from build123d import *

# Parameters (mm, degrees)
SKETCH_1_W               = 20
SKETCH_1_H               = 20
SKETCH_1_W_2             = 16
SKETCH_1_H_2             = 16
EXTRUDE_1_DEPTH          = 560
SKETCH_3_R               = 2.2
CUT_EXTRUDE_2_DEPTH      = 560
SKETCH_4_R               = 2.2
CUT_EXTRUDE_3_DEPTH      = 560
SKETCH_7_W               = 41.109335544
SKETCH_7_H               = 41.63539172
CUT_EXTRUDE_7_DEPTH      = 40
SKETCH_8_W               = 53.430317452
SKETCH_8_H               = 33.679555816
CUT_EXTRUDE_8_DEPTH      = 40
SKETCH_9_R               = 1
CUT_EXTRUDE_9_DEPTH      = 10
SKETCH_10_R              = 1
CUT_EXTRUDE_10_DEPTH     = 10
SKETCH_11_R              = 2.1
CUT_EXTRUDE_11_DEPTH     = 21
SKETCH_12_R              = 6
CUT_EXTRUDE_12_DEPTH     = 10
SKETCH_15_R              = 2.1
CUT_EXTRUDE_16_DEPTH     = 21
SKETCH_16_R              = 6
CUT_EXTRUDE_17_DEPTH     = 10
M4X0_7_6_D               = 3.3
M4X0_7_6_DEPTH           = 11.5
M4X0_7_6_TIP             = 0.991420021
M4X0_7_7_D               = 3.3
M4X0_7_7_DEPTH           = 11.5
M4X0_7_7_TIP             = 0.991420021
M4X0_7_7_ON_FACE_2_D     = 3.3
M4X0_7_7_ON_FACE_2_DEPTH = 11.5
M4X0_7_7_ON_FACE_2_TIP   = 0.991420021
SKETCH_26_R              = 1
CUT_EXTRUDE_18_DEPTH     = 10
M4X0_7_9_D               = 3.3
M4X0_7_9_DEPTH           = 11.5
M4X0_7_9_TIP             = 0.991420021


with BuildPart() as part:
    # ｽｹｯﾁ1 → ﾎﾞｽ - 押し出し1 (new body)
    with BuildSketch(Plane.XY):
        Rectangle(SKETCH_1_W, SKETCH_1_H)
        Rectangle(SKETCH_1_W_2, SKETCH_1_H_2, mode=Mode.SUBTRACT)
    extrude(amount=EXTRUDE_1_DEPTH)

    # ｽｹｯﾁ3 → ｶｯﾄ - 押し出し2 (cut)
    with BuildSketch(Plane(origin=(10, 0, 0), x_dir=(0, 0, -1), z_dir=(1, 0, 0))):
        with Locations((-530, 0)):
            Circle(SKETCH_3_R)
        with Locations((-30, 0)):
            Circle(SKETCH_3_R)
    extrude(amount=-CUT_EXTRUDE_2_DEPTH, mode=Mode.SUBTRACT)

    # ｽｹｯﾁ4 → ｶｯﾄ - 押し出し3 (cut)
    with BuildSketch(Plane(origin=(0, 10, 0), x_dir=(1, 0, 0), z_dir=(0, 1, 0))):
        with Locations((0, -550)):
            Circle(SKETCH_4_R)
        with Locations((0, -10)):
            Circle(SKETCH_4_R)
    extrude(amount=-CUT_EXTRUDE_3_DEPTH, mode=Mode.SUBTRACT)

    # ｽｹｯﾁ7 → ｶｯﾄ - 押し出し7 (cut)
    with BuildSketch(Plane(origin=(0, 0, 0), x_dir=(-1, 0, 0), z_dir=(0, 0, -1))):
        Rectangle(SKETCH_7_W, SKETCH_7_H)
    extrude(amount=-CUT_EXTRUDE_7_DEPTH, mode=Mode.SUBTRACT)

    # ｽｹｯﾁ8 → ｶｯﾄ - 押し出し8 (cut)
    with BuildSketch(Plane.XY.offset(560)):
        Rectangle(SKETCH_8_W, SKETCH_8_H)
    extrude(amount=-CUT_EXTRUDE_8_DEPTH, mode=Mode.SUBTRACT)

    # ｽｹｯﾁ9 → ｶｯﾄ - 押し出し9 (cut)
    with BuildSketch(Plane.ZY.offset(10)):
        with Locations((510, 0)):
            Circle(SKETCH_9_R)
        with Locations((490, 0)):
            Circle(SKETCH_9_R)
    extrude(amount=-CUT_EXTRUDE_9_DEPTH, mode=Mode.SUBTRACT)

    # ｽｹｯﾁ10 → ｶｯﾄ - 押し出し10 (cut)
    with BuildSketch(Plane.ZY.offset(10)):
        with Locations((50, 0)):
            Circle(SKETCH_10_R)
        with Locations((70, 0)):
            Circle(SKETCH_10_R)
    extrude(amount=-CUT_EXTRUDE_10_DEPTH, mode=Mode.SUBTRACT)

    # ｽｹｯﾁ11 → ｶｯﾄ - 押し出し11 (cut, through all)
    with BuildSketch(Plane(origin=(0, 10, 0), x_dir=(1, 0, 0), z_dir=(0, 1, 0))):
        with Locations((0, -60)):
            Circle(SKETCH_11_R)
        with Locations((0, -132)):
            Circle(SKETCH_11_R)
        with Locations((0, -204)):
            Circle(SKETCH_11_R)
    extrude(amount=-CUT_EXTRUDE_11_DEPTH, mode=Mode.SUBTRACT)

    # ｽｹｯﾁ12 → ｶｯﾄ - 押し出し12 (cut)
    with BuildSketch(Plane(origin=(0, 10, 0), x_dir=(1, 0, 0), z_dir=(0, 1, 0))):
        with Locations((0, -60)):
            Circle(SKETCH_12_R)
        with Locations((0, -132)):
            Circle(SKETCH_12_R)
        with Locations((0, -204)):
            Circle(SKETCH_12_R)
    extrude(amount=-CUT_EXTRUDE_12_DEPTH, mode=Mode.SUBTRACT)

    # ｽｹｯﾁ15 → ｶｯﾄ - 押し出し16 (cut, through all)
    with BuildSketch(Plane(origin=(0, 10, 0), x_dir=(1, 0, 0), z_dir=(0, 1, 0))):
        with Locations((0, -326)):
            Circle(SKETCH_15_R)
    extrude(amount=-CUT_EXTRUDE_16_DEPTH, mode=Mode.SUBTRACT)

    # ｽｹｯﾁ16 → ｶｯﾄ - 押し出し17 (cut)
    with BuildSketch(Plane(origin=(0, 10, 0), x_dir=(1, 0, 0), z_dir=(0, 1, 0))):
        with Locations((0, -326)):
            Circle(SKETCH_16_R)
    extrude(amount=-CUT_EXTRUDE_17_DEPTH, mode=Mode.SUBTRACT)

    # M4x0.7 ねじ穴6
    with Locations(Plane(origin=(-10, 0, 70), x_dir=(0, -1, 0), z_dir=(-1, 0, 0))):
        with Locations((0, 0), (0, -20)):
            Hole(M4X0_7_6_D / 2, depth=M4X0_7_6_DEPTH)
            with Locations((0, 0, -(M4X0_7_6_DEPTH + M4X0_7_6_TIP / 2))):  # 118° drill point
                Cone(0, M4X0_7_6_D / 2, M4X0_7_6_TIP, mode=Mode.SUBTRACT)

    # M4x0.7 ねじ穴7
    with Locations(Plane(origin=(-8, 0, 490), x_dir=(0, 0, 1), z_dir=(1, 0, 0))):
        with Locations((0, 0)):
            Hole(M4X0_7_7_D / 2, depth=M4X0_7_7_DEPTH)
            with Locations((0, 0, -(M4X0_7_7_DEPTH + M4X0_7_7_TIP / 2))):  # 118° drill point
                Cone(0, M4X0_7_7_D / 2, M4X0_7_7_TIP, mode=Mode.SUBTRACT)

    # M4x0.7 ねじ穴7 on face 2
    with Locations(Plane(origin=(-10, 0, 510), x_dir=(0, 0, 1), z_dir=(1, 0, 0))):
        with Locations((0, 0)):
            Hole(M4X0_7_7_ON_FACE_2_D / 2, depth=M4X0_7_7_ON_FACE_2_DEPTH)
            with Locations((0, 0, -(M4X0_7_7_ON_FACE_2_DEPTH + M4X0_7_7_ON_FACE_2_TIP / 2))):  # 118° drill point
                Cone(0, M4X0_7_7_ON_FACE_2_D / 2, M4X0_7_7_ON_FACE_2_TIP, mode=Mode.SUBTRACT)

    # ｽｹｯﾁ26 → ｶｯﾄ - 押し出し18 (cut)
    with BuildSketch(Plane(origin=(10, 0, 0), x_dir=(0, 0, -1), z_dir=(1, 0, 0))):
        with Locations((-446, -5)):
            Circle(SKETCH_26_R)
        with Locations((-412, -5)):
            Circle(SKETCH_26_R)
    extrude(amount=-CUT_EXTRUDE_18_DEPTH, mode=Mode.SUBTRACT)

    # M4x0.7 ねじ穴9
    with Locations(Plane(origin=(10, -5, 446), x_dir=(0, 0, 1), z_dir=(1, 0, 0))):
        with Locations((0, 0), (-34, 0)):
            Hole(M4X0_7_9_D / 2, depth=M4X0_7_9_DEPTH)
            with Locations((0, 0, -(M4X0_7_9_DEPTH + M4X0_7_9_TIP / 2))):  # 118° drill point
                Cone(0, M4X0_7_9_D / 2, M4X0_7_9_TIP, mode=Mode.SUBTRACT)


solid = part.part
For this review, take the finished solid that the model builds, in its own axes (mm). A direction names the side the tool comes from. Coordinates: 2 decimals unless noted, no trailing zeros. Order: outer loops, then holes, each group sorted by start corner. A loop starts at its lowest first (then second) coordinate and runs counter-clockwise, first axis right, second up. Notation, with made-up numbers: (67, -28) -> (110, -28) arc R25 cw to (110, 3) -> close; hole circle Ø7 at (-23.5, 82). An arc over 180 degrees is marked (long way). Return JSON: item names as keys, results as strings.
1. The part is to be moulded in two halves that separate along Y. For faces 4 (the flat face through (0, 8, 277)), 5 (the flat face through (0, -10, 277)), 6 (the flat face through (-9, 0, 520)), 7 (the flat face through (0, 10, 277)), say which applies: +Y half, -Y half, draft (parallel to the pull), parting line (faces both ways), or undercut.
Answer block:
{"face 4": "undercut", "face 5": "-Y half", "face 6": "draft", "face 7": "+Y half"}
2. Machinability: for faces 1 (the flat face through (9, 0, 40)), 2 (the flat face through (0, -8, 277)), 3 (the cylindrical face through (3.226, 9.014, 320.941)), which of the approach directions +Z, -Z, +X, -X, +Y, -Y give a long, thin tool a straight path to every point of the face, cutting with its end or side? Answer none if there is none.
Answer block:
{"face 1": "-Z, +X, -X, +Y, -Y", "face 2": "+Z, -Z", "face 3": "+Y"}
3. We need section A-A on z = 257.5. Write out the cut boundary in (x, y), and give its area (3 significant figures).
Answer block:
{"outline": "(-10, -10) -> (10, -10) -> (10, 10) -> (-10, 10) -> close; hole (-8, -8) -> (8, -8) -> (8, 8) -> (-8, 8) -> close", "area": "144 mm²"}
4. For pin 1 Ø4 at (y, z) = (0, 510) entering from -X; pin 2 Ø2.5 at (y, z) = (-5, 446) entering from +X; pin 3 Ø5 at (x, z) = (0.5, 201) entering from +Y, all flat-tipped, find the tip position at first contact; note any pin that passes through.
Answer block:
{"pin 1": "x = -10", "pin 2": "x = -8", "pin 3": "y = -8"}
5. For line 1 (X direction, y = -2, z = 186); line 2 (X direction, y = -9.55, z = 132), list the stretches that pass through material, from the lowest coordinate up. Write a range as from..to.
Answer block:
{"line 1": "-10..-8, 8..10", "line 2": "-10..-2.1, 2.1..10"}
